The model under review builds one solid part; all positions refer to its coordinate system, in mm. A direction names the side the tool comes from. Give positions to 0.01 mm unless a question says otherwise; leave off trailing zeros. Order: outer loops, then holes, each group sorted by start corner. A loop starts at its lowest first (then second) coordinate and runs counter-clockwise, first axis right, second up. Notation, with made-up numbers: (63, 38.5) -> (67, 38.5) arc R27 cw to (67, 65.5) -> close; hole circle Ø8 at (64, -11). An arc over 180 degrees is marked (long way). Answer as a JSON object with one key per item and string values. Group by question number.
from build123d import *

# Parameters (mm, degrees)
SKETCH1_W                = 80
SKETCH1_H                = 80
BOSS_EXTRUDE1_DEPTH      = 3.175
CUT_EXTRUDE1_START       = -3.175
CUT_EXTRUDE1_OUTLINE_W   = 3.175
CUT_EXTRUDE1_OUTLINE_H   = 4.91
CUT_EXTRUDE1_OUTLINE_W_2 = 5.333333333
CUT_EXTRUDE1_OUTLINE_H_2 = 3.175
CUT_EXTRUDE1_OUTLINE_W_3 = 5.333333334
CUT_EXTRUDE1_DEPTH       = 3.175
SKETCH3_R                = 1.15
CUT_EXTRUDE2_DEPTH       = 57.657573413


# Read off the part's stored shape, not the designer's step: Cut-Extrude1
with BuildPart() as part:
    # Sketch1 → Boss-Extrude1 (new body)
    with BuildSketch(Plane.XY):
        Rectangle(SKETCH1_W, SKETCH1_H)
    extrude(amount=BOSS_EXTRUDE1_DEPTH)

    # Cut-Extrude1 outline → Cut-Extrude1 (cut)
    with BuildSketch(Plane.XY.offset(3.175).offset(CUT_EXTRUDE1_START)):
        with Locations((-38.4125, 29.46)):
            Rectangle(CUT_EXTRUDE1_OUTLINE_W, CUT_EXTRUDE1_OUTLINE_H)
        with Locations((-37.333333334, 38.4125)):
            Rectangle(CUT_EXTRUDE1_OUTLINE_W_2, CUT_EXTRUDE1_OUTLINE_H_2)
        with Locations((-38.4125, 19.64)):
            Rectangle(CUT_EXTRUDE1_OUTLINE_W, CUT_EXTRUDE1_OUTLINE_H)
        with Locations((-38.4125, 9.82)):
            Rectangle(CUT_EXTRUDE1_OUTLINE_W, CUT_EXTRUDE1_OUTLINE_H)
        with Locations((-26.666666666, 38.4125)):
            Rectangle(CUT_EXTRUDE1_OUTLINE_W_2, CUT_EXTRUDE1_OUTLINE_H_2)
        with Locations((-38.4125, 0)):
            Rectangle(CUT_EXTRUDE1_OUTLINE_W, CUT_EXTRUDE1_OUTLINE_H)
        with Locations((-16, 38.4125)):
            Rectangle(CUT_EXTRUDE1_OUTLINE_W_3, CUT_EXTRUDE1_OUTLINE_H_2)
        with Locations((-38.4125, -9.82)):
            Rectangle(CUT_EXTRUDE1_OUTLINE_W, CUT_EXTRUDE1_OUTLINE_H)
        with Locations((-5.333333334, 38.4125)):
            Rectangle(CUT_EXTRUDE1_OUTLINE_W_2, CUT_EXTRUDE1_OUTLINE_H_2)
        with Locations((-38.4125, -19.64)):
            Rectangle(CUT_EXTRUDE1_OUTLINE_W, CUT_EXTRUDE1_OUTLINE_H)
        with Locations((5.333333334, 38.4125)):
            Rectangle(CUT_EXTRUDE1_OUTLINE_W_2, CUT_EXTRUDE1_OUTLINE_H_2)
        with Locations((-38.4125, -29.46)):
            Rectangle(CUT_EXTRUDE1_OUTLINE_W, CUT_EXTRUDE1_OUTLINE_H)
        with Locations((16, 38.4125)):
            Rectangle(CUT_EXTRUDE1_OUTLINE_W_3, CUT_EXTRUDE1_OUTLINE_H_2)
        with Locations((-37.333333334, -38.4125)):
            Rectangle(CUT_EXTRUDE1_OUTLINE_W_2, CUT_EXTRUDE1_OUTLINE_H_2)
        with Locations((26.666666666, 38.4125)):
            Rectangle(CUT_EXTRUDE1_OUTLINE_W_2, CUT_EXTRUDE1_OUTLINE_H_2)
        with Locations((37.333333334, 38.4125)):
            Rectangle(CUT_EXTRUDE1_OUTLINE_W_2, CUT_EXTRUDE1_OUTLINE_H_2)
        with Locations((-26.666666666, -38.4125)):
            Rectangle(CUT_EXTRUDE1_OUTLINE_W_2, CUT_EXTRUDE1_OUTLINE_H_2)
        with Locations((-16, -38.4125)):
            Rectangle(CUT_EXTRUDE1_OUTLINE_W_3, CUT_EXTRUDE1_OUTLINE_H_2)
        with Locations((38.4125, 29.46)):
            Rectangle(CUT_EXTRUDE1_OUTLINE_W, CUT_EXTRUDE1_OUTLINE_H)
        with Locations((-5.333333334, -38.4125)):
            Rectangle(CUT_EXTRUDE1_OUTLINE_W_2, CUT_EXTRUDE1_OUTLINE_H_2)
        with Locations((38.4125, 19.64)):
            Rectangle(CUT_EXTRUDE1_OUTLINE_W, CUT_EXTRUDE1_OUTLINE_H)
        with Locations((5.333333334, -38.4125)):
            Rectangle(CUT_EXTRUDE1_OUTLINE_W_2, CUT_EXTRUDE1_OUTLINE_H_2)
        with Locations((38.4125, 9.82)):
            Rectangle(CUT_EXTRUDE1_OUTLINE_W, CUT_EXTRUDE1_OUTLINE_H)
        with Locations((16, -38.4125)):
            Rectangle(CUT_EXTRUDE1_OUTLINE_W_3, CUT_EXTRUDE1_OUTLINE_H_2)
        with Locations((38.4125, 0)):
            Rectangle(CUT_EXTRUDE1_OUTLINE_W, CUT_EXTRUDE1_OUTLINE_H)
        with Locations((26.666666666, -38.4125)):
            Rectangle(CUT_EXTRUDE1_OUTLINE_W_2, CUT_EXTRUDE1_OUTLINE_H_2)
        with Locations((38.4125, -9.82)):
            Rectangle(CUT_EXTRUDE1_OUTLINE_W, CUT_EXTRUDE1_OUTLINE_H)
        with Locations((37.333333334, -38.4125)):
            Rectangle(CUT_EXTRUDE1_OUTLINE_W_2, CUT_EXTRUDE1_OUTLINE_H_2)
        with Locations((38.4125, -19.64)):
            Rectangle(CUT_EXTRUDE1_OUTLINE_W, CUT_EXTRUDE1_OUTLINE_H)
        with Locations((38.4125, -29.46)):
            Rectangle(CUT_EXTRUDE1_OUTLINE_W, CUT_EXTRUDE1_OUTLINE_H)
    extrude(amount=CUT_EXTRUDE1_DEPTH, mode=Mode.SUBTRACT)

    # Sketch3 → Cut-Extrude2 (cut, through all)
    with BuildSketch(Plane(origin=(0, 0, 0), x_dir=(-1, 0, 0), z_dir=(0, 0, -1))):
        with Locations((-10.28, -6.975)):
            Circle(SKETCH3_R)
        with Locations((-10.3, -29.875)):
            Circle(SKETCH3_R)
        with Locations(Location((10.3, -29.875, 0), (0, 0, 180))):
            Circle(SKETCH3_R)
        with Locations(Location((10.28, -6.975, 0), (0, 0, 180))):
            Circle(SKETCH3_R)
        Polygon((6, -4.825), (6, -9.125), (13.65, -9.125), (13.65, -28.125), (-13.65, -28.125), (-13.65, -9.125), (-6, -9.125), (-6, -4.825), align=None)
    extrude(amount=-CUT_EXTRUDE2_DEPTH, mode=Mode.SUBTRACT)


solid = part.part
1. For probe 1 along Y at (x, z) = (10.28, 1.2) (3 decimals); probe 2 along X at (y, z) = (-8.5, 0.2) (3 decimals); probe 3 along X at (y, z) = (-21, 1.4) (3 decimals), list the stretches that pass through material, from the lowest coordinate up. Write a range as [from, to].
2. Take a section at A-A on x = 10.28. Give the boundary of the cut face in (y, z) (3 decimals), plus the area to 3 significant figures.
3. Machinability: for faces 1 (the flat face through (-29.333, -38, 2)), 2 (the flat face through (38, -2.455, 2)), 3 (the flat face through (-38, -22.095, 2)), 4 (the flat face through (13.333, 38, 2)), which of the approach directions +Z, -Z, +X, -X, +Y, -Y give a long, thin tool a straight path to every point of the face, cutting with its end or side? Answer none if there is none.
4. Take a section at B-B on x = 26.5. Give the boundary of the cut face in (y, z) (3 decimals).
5. Draft analysis for pull direction X (two halves, no side actions). For faces 5 (the flat face through (36.825, 10, 2)), 6 (the flat face through (38, 2.455, 2)), 7 (the flat face through (-29.333, 38, 2)), state which applies: pulls with the +X half, pulls with the -X half, needs draft (parallel to the pull), parting line crosses it, or undercut.
6. For pin 1 (1 mm diameter, centred on y = 0, z = 2, fed in from -X) (3 decimals); pin 2 (1.6 mm diameter, centred on x = -37.5, z = 1, fed in from -Y) (3 decimals); pin 3 (1.6 mm diameter, centred on x = -16.5, z = 1, fed in from +Y) (3 decimals), all flat-tipped, find the tip position at first contact; note any pin that passes through.
7. Take a section at C-C on z = 2.5. State how many separate pieces and enclosed holes the cut face has, plus the area to 3 significant figures.
Checks:
{
 "1": {"probe 1": "y = [-40, -31.025], [-28.725, -28.125], [-9.125, -8.125], [-5.825, 40]", "probe 2": "x = [-36.825, -6], [6, 36.825]", "probe 3": "x = [-36.825, -13.65], [13.65, 36.825]"},
 "2": {"outline": "(-40, 0) -> (-31.025, 0) -> (-31.025, 3.175) -> (-40, 3.175) -> close; (-28.725, 0) -> (-28.125, 0) -> (-28.125, 3.175) -> (-28.725, 3.175) -> close; (-9.125, 0) -> (-8.125, 0) -> (-8.125, 3.175) -> (-9.125, 3.175) -> close; (-5.825, 0) -> (40, 0) -> (40, 3.175) -> (-5.825, 3.175) -> close", "area": "179 mm2"},
 "3": {"face 1": "+Z, -Z, -Y", "face 2": "+Z, -Z, +X", "face 3": "+Z, -Z, -X", "face 4": "+Z, -Z, +Y"},
 "4": {"outline": "(-36.825, 0) -> (36.825, 0) -> (36.825, 3.175) -> (-36.825, 3.175) -> close"},
 "5": {"face 5": "pulls with the +X half", "face 6": "needs draft", "face 7": "undercut"},
 "6": {"pin 1": "stops at x = -36.825", "pin 2": "stops at y = -36.825", "pin 3": "stops at y = 36.825"},
 "7": {"separate pieces": "1", "enclosed holes": "5", "area": "5,320 mm2"}
}
